Source: three-view drawing plus pictorial views. Frame: mm from the lowest corner of the part. Round coordinates to 2 decimals unless told otherwise and drop trailing zeros. Write each loop counter-clockwise with the first axis right and the second up, starting at its lowest first coordinate (ties: lowest second). Pieces come first, ordered by that corner, then holes.
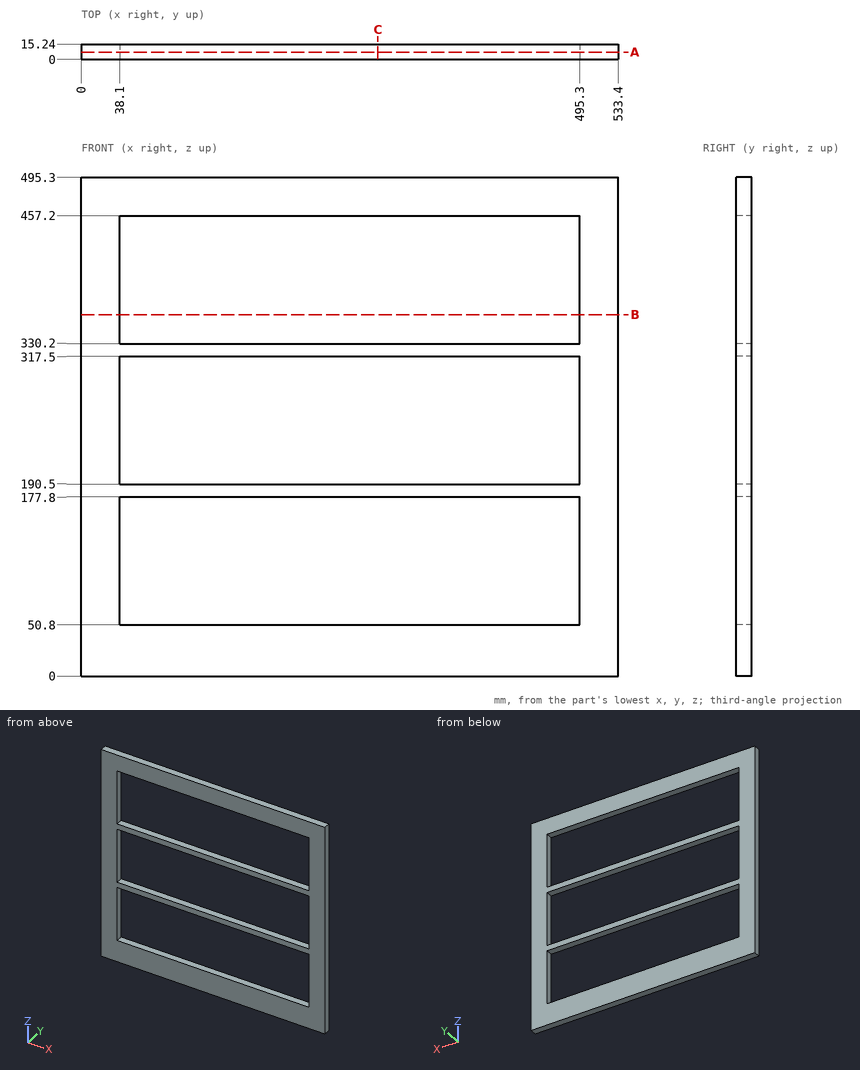
1) Line query: probe 1 along Z at (x, y) = (424, 11.25); probe 2 along X at (y, z) = (9.5, 406). Output: solid intervals per line, ascending.
2) Section C-C on x = 294.5. Output: boundary loops of the cut face in (y, z).
3) Section A-A on y = 7.25. Output: boundary loops of the cut face in (x, z), plus the area to 3 significant figures.
4) First-contact query: P1, Ø2, axis at y = 3.5, z = 205.5, coming from the -X side. Flat tip, straight axial feed; report the tip coordinate or a pass-through.
5) Section B-B on z = 359. Output: boundary loops of the cut face in (x, y).
Filled in:
1. probe 1: z = 0 to 50.8, 177.8 to 190.5, 317.5 to 330.2, 457.2 to 495.3
1. probe 2: x = 0 to 38.1, 495.3 to 533.4
2. outline: (0, 0) - (15.24, 0) - (15.24, 50.8) - (0, 50.8) - close; (0, 177.8) - (15.24, 177.8) - (15.24, 190.5) - (0, 190.5) - close; (0, 317.5) - (15.24, 317.5) - (15.24, 330.2) - (0, 330.2) - close; (0, 457.2) - (15.24, 457.2) - (15.24, 495.3) - (0, 495.3) - close
3. outline: (0, 0) - (533.4, 0) - (533.4, 495.3) - (0, 495.3) - close; hole (38.1, 50.8) - (495.3, 50.8) - (495.3, 177.8) - (38.1, 177.8) - close; hole (38.1, 190.5) - (495.3, 190.5) - (495.3, 317.5) - (38.1, 317.5) - close; hole (38.1, 330.2) - (495.3, 330.2) - (495.3, 457.2) - (38.1, 457.2) - close
3. area: 90,000 mm2
4. P1: stops at x = 0
5. outline: (0, 0) - (38.1, 0) - (38.1, 15.24) - (0, 15.24) - close; (495.3, 0) - (533.4, 0) - (533.4, 15.24) - (495.3, 15.24) - close
